Design review of the part built by this model. Coordinates are the model's own, in mm. Coordinates: 2 decimals unless noted, no trailing zeros. Write each loop counter-clockwise with the first axis right and the second up, starting at its lowest first coordinate (ties: lowest second). Pieces come first, ordered by that corner, then holes. Notation, with made-up numbers: M -4.5,-19 L 18.5,-19 A21 ccw 18.5,18 Z; hole C 87.25,42.25 d9. An arc over 180 degrees is marked long. Write each question's results on one line, items separated by ' | '. Start each with the question number.
```python
from build123d import *

# Parameters (mm, degrees)
F0_W     = 79.0346935391
F0_H     = 56.1182498932
F1_DEPTH = 50.8
F2_R     = 5.08
F3_R     = 8.9977946324
F4_DEPTH = 56.1192498932


with BuildPart() as f1:
    # F0 (on Front) → F1 (new body)
    with BuildSketch(Plane.XZ):
        with Locations((10.1048909128, 1.1728554964)):
            Rectangle(F0_W, F0_H)
    extrude(amount=F1_DEPTH)

    # F2
    f2_edges = [f1.edges().sort_by_distance(p)[0] for p in [
        (10.104891, -50.8, -26.886269),
        (-29.412456, -50.8, 1.172855),
        (10.104891, -50.8, 29.23198),
        (49.622238, -50.8, 1.172855),
        (49.622238, -25.4, -26.886269),
        (10.104891, 0, -26.886269),
        (-29.412456, -25.4, -26.886269),
        (49.622238, -25.4, 29.23198),
        (10.104891, 0, 29.23198),
        (-29.412456, 0, 1.172855),
        (49.622238, 0, 1.172855),
        (-29.412456, -25.4, 29.23198),
    ]]
    fillet(f2_edges, radius=F2_R)

    # F3 (on face) → F4 (cut, through all)
    with BuildSketch(Plane.XY.offset(29.231980443)):
        with Locations((9.6274446696, -24.0743868053)):
            Circle(F3_R)
    extrude(amount=-F4_DEPTH, mode=Mode.SUBTRACT)


solid = f1.part
```
Item 1: Draft analysis for pull direction X (two halves, no side actions). For faces 1 (the cylindrical face through (-27.964, -25.684, 27.704)), 2 (the cylindrical face through (2.49, -29.55, 1.57)), 3 (the cylindrical face through (48.09, -25.68, -25.44)), 4 (the flat face through (10, 0, 1)), state which applies: released by +X, released by -X, zero draft, split by the parting line, or undercut.
Item 2: We need section A-A on y = -25. State the section outline as (x, z) points, then the cut area to 3 significant figures.
Item 3: We need section D-D on z = 26. State the section outline as (x, y) points, then the cut area to 3 significant figures.
Item 4: We need section B-B on z = -16. State the section outline as (x, y) points.
Item 5: Insertion check: pin 1 Ø11 at (x, y) = (9.63, -24.07) entering from -Z. The pin has a flat end and moves straight along its axis. Give the tip position at first contact, or say it passes through.
Item 6: Wall thickness on L1, parallel to Z at x = 39.5, y = -46; L2, parallel to X at y = -17, z = -12; L3, parallel to X at y = -16, z = -1: over which ranges is each line inside the solid? List them lowest first.
Item 7: We need section C-C on x = 5.5. State the section outline as (y, z) points, then the cut area to 3 significant figures.
Answer:
1) face 1: released by -X | face 2: undercut | face 3: released by +X | face 4: zero draft
2) outline: M -29.41,-21.81 A5.08 ccw -24.33,-26.89 L 0.68,-26.89 L 0.68,29.23 L -24.33,29.23 A5.08 ccw -29.41,24.15 Z; M 18.58,-26.89 L 44.54,-26.89 A5.08 ccw 49.62,-21.81 L 49.62,24.15 A5.08 ccw 44.54,29.23 L 18.58,29.23 Z | area: 3,410 mm^2
3) outline: M -29.06,-45.72 A4.73 ccw -24.33,-50.45 L 44.54,-50.45 A4.73 ccw 49.27,-45.72 L 49.27,-5.08 A4.73 ccw 44.54,-0.35 L -24.33,-0.35 A4.73 ccw -29.06,-5.08 Z; hole C 9.63,-24.07 d18 | area: 3,650 mm^2
4) outline: M -29.41,-45.72 A5.08 ccw -24.33,-50.8 L 44.54,-50.8 A5.08 ccw 49.62,-45.72 L 49.62,-5.08 A5.08 ccw 44.54,0 L -24.33,0 A5.08 ccw -29.41,-5.08 Z; hole C 9.63,-24.07 d18
5) pin 1: passes through
6) L1: z = -26.88 to 29.22 | L2: x = -29.41 to 4.07, 15.19 to 49.62 | L3: x = -29.41 to 5.66, 13.6 to 49.62
7) outline: M -50.8,-21.81 A5.08 ccw -45.72,-26.89 L -32.07,-26.89 L -32.07,29.23 L -45.72,29.23 A5.08 ccw -50.8,24.15 Z; M -16.08,-26.89 L -5.08,-26.89 A5.08 ccw 0,-21.81 L 0,24.15 A5.08 ccw -5.08,29.23 L -16.08,29.23 Z | area: 1,930 mm^2
